```python
from build123d import *

# Parameters (mm, degrees)
SKETCH1_W           = 271.78
SKETCH1_H           = 121.92
SKETCH1_R           = 2.54
BOSS_EXTRUDE1_DEPTH = 5.08
FILLET1_R           = 6.35
SKETCH3_W           = 17.4625
SKETCH3_H           = 5.08
CUT_EXTRUDE2_DEPTH  = 7.62
FILLET2_R           = 11.43


with BuildPart() as part:
    # Sketch1 → Boss-Extrude1 (new body)
    with BuildSketch(Plane(origin=(0, 0, 0), x_dir=(1, 0, 0), z_dir=(0, 1, 0))):
        Rectangle(SKETCH1_W, SKETCH1_H)
        with Locations((-50.8, -38.1)):
            Circle(SKETCH1_R, mode=Mode.SUBTRACT)
        Polygon((-125.73, 42.241214341), (-94.577104423, 0), (-125.73, -42.241214341), align=None, mode=Mode.SUBTRACT)
        Polygon((-88.265, -8.558785659), (-57.112104423, -50.8), (-119.417895577, -50.8), align=None, mode=Mode.SUBTRACT)
        Polygon((-55.88, -35.353078748), (-81.952895577, 0), (-55.88, 35.353078748), align=None, mode=Mode.SUBTRACT)
        Polygon((-35.524026052, -50.8), (37.465, -8.791927452), (110.454026052, -50.8), align=None, mode=Mode.SUBTRACT)
        Polygon((22.189026052, 0), (-45.72, -39.084331541), (-45.72, 39.084331541), align=None, mode=Mode.SUBTRACT)
        Polygon((-57.112104423, 50.8), (-88.265, 8.558785659), (-119.417895577, 50.8), align=None, mode=Mode.SUBTRACT)
        with Locations((-50.8, 38.1)):
            Circle(SKETCH1_R, mode=Mode.SUBTRACT)
        Polygon((52.740973948, 0), (125.73, 42.008072548), (125.73, -42.008072548), align=None, mode=Mode.SUBTRACT)
        Polygon((110.454026052, 50.8), (37.465, 8.791927452), (-35.524026052, 50.8), align=None, mode=Mode.SUBTRACT)
    extrude(amount=BOSS_EXTRUDE1_DEPTH)

    # Fillet1
    fillet1_edges = [part.edges().sort_by_distance(p)[0] for p in [
        (-35.524026052, 2.54, 50.8),
        (37.465, 2.54, 8.791927452),
        (125.73, 2.54, 42.008072548),
        (125.73, 2.54, -42.008072548),
        (52.740973948, 2.54, 0),
        (-45.72, 2.54, 39.084331541),
        (22.189026052, 2.54, 0),
        (-45.72, 2.54, -39.084331541),
        (-35.524026052, 2.54, -50.8),
        (37.465, 2.54, -8.791927452),
        (-125.73, 2.54, -42.241214341),
        (-125.73, 2.54, 42.241214341),
        (-94.577104423, 2.54, 0),
        (-57.112104423, 2.54, -50.8),
        (-119.417895577, 2.54, -50.8),
        (-88.265, 2.54, -8.558785659),
        (-119.417895577, 2.54, 50.8),
        (-57.112104423, 2.54, 50.8),
        (-88.265, 2.54, 8.558785659),
        (-55.88, 2.54, 35.353078748),
        (-55.88, 2.54, -35.353078748),
        (-81.952895577, 2.54, 0),
    ]]
    fillet(fillet1_edges, radius=FILLET1_R)

    # Sketch3 → Cut-Extrude2 (cut)
    with BuildSketch(Plane(origin=(0, 5.08, 0), x_dir=(1, 0, 0), z_dir=(0, 1, 0))):
        with Locations((92.23375, 58.42)):
            Rectangle(SKETCH3_W, SKETCH3_H)
        with Locations((127.15875, 58.42)):
            Rectangle(SKETCH3_W, SKETCH3_H)
        with Locations((92.23375, -58.42)):
            Rectangle(SKETCH3_W, SKETCH3_H)
        with Locations((127.15875, -58.42)):
            Rectangle(SKETCH3_W, SKETCH3_H)
    extrude(amount=-CUT_EXTRUDE2_DEPTH, mode=Mode.SUBTRACT)

    # Fillet2
    fillet2_edges = [part.edges().sort_by_distance(p)[0] for p in [
        (110.454026052, 2.54, 50.8),
        (110.454026052, 2.54, -50.8),
    ]]
    fillet(fillet2_edges, radius=FILLET2_R)


solid = part.part
```
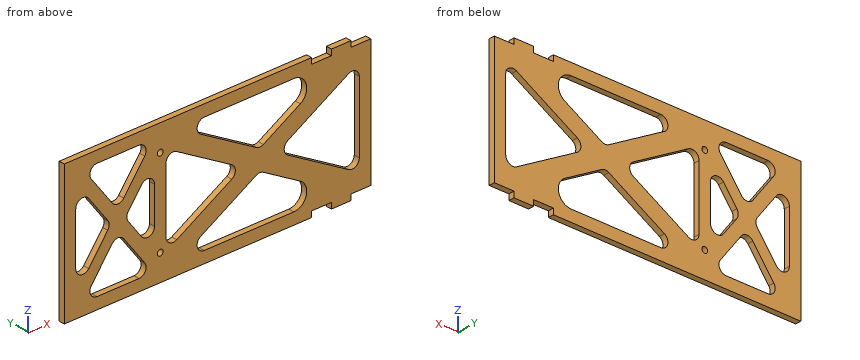
Design review of the part built by this model. Coordinates are the model's own, in mm. Coordinates: 2 decimals unless noted, no trailing zeros. Order: outer loops, then holes, each group sorted by start corner. A loop starts at its lowest first (then second) coordinate and runs counter-clockwise, first axis right, second up. Notation, with made-up numbers: (34.25, -21.75) -> (88.25, -21.75) arc R20 cw to (88.25, 15.25) -> close; hole circle Ø8 at (-6.5, 53.25). An arc over 180 degrees is marked (long way). One line per item, written item: value. Start each with the question number.
Q1. Take a section at B-B, the plane z = 0.5. State the section outline as (x, y) points, then the cut area to 3 significant figures.
Q2. Take a section at A-A, the plane x = -50.8. State the section outline as (y, z) points.
Q3. For probe 1 along Z at (x, y) = (-50.8, 1.85); probe 2 along X at (y, z) = (2.55, 29.5); probe 3 along Z at (x, y) = (-109.5, 0.35), list the stretches that pass through material, from the lowest coordinate up.
Q4. Insertion check: pin 1 Ø1.5 at (y, z) = (2, 58.5) entering from +X; pin 2 Ø1.5 at (x, y) = (124.5, 3) entering from -Z. Each pin has a flat end and moves straight along its axis. Give the tip position at first contact, or say it passes through.
Q5. Take a section at C-C, the plane y = 1.85. Give the number of separate pieces and of enclosed holes in the cut face, then the cut area to 3 significant figures.
Values follow:
1. outline: (-135.89, 0) -> (-125.73, 0) -> (-125.73, 5.08) -> (-135.89, 5.08) -> close; (-96.14, 0) -> (-80.39, 0) -> (-80.39, 5.08) -> (-96.14, 5.08) -> close; (-55.88, 0) -> (-45.72, 0) -> (-45.72, 5.08) -> (-55.88, 5.08) -> close; (15.79, 0) -> (59.14, 0) -> (59.14, 5.08) -> (15.79, 5.08) -> close; (125.73, 0) -> (135.89, 0) -> (135.89, 5.08) -> (125.73, 5.08) -> close
1. area: 455 mm2
2. outline: (0, -60.96) -> (5.08, -60.96) -> (5.08, -40.64) -> (0, -40.64) -> close; (0, -35.56) -> (5.08, -35.56) -> (5.08, 35.56) -> (0, 35.56) -> close; (0, 40.64) -> (5.08, 40.64) -> (5.08, 60.96) -> (0, 60.96) -> close
3. probe 1: z = -60.96 to -40.64, -35.56 to 35.56, 40.64 to 60.96
3. probe 2: x = -135.89 to -103.71, -72.82 to -45.56, -29.07 to 1.48, 73.44 to 104, 125.73 to 135.89
3. probe 3: z = -60.96 to -50.22, -37.35 to -20.23, 20.23 to 37.35, 50.22 to 60.96
4. pin 1: stops at x = 118.43
4. pin 2: stops at z = -55.88
5. separate pieces: 1
5. enclosed holes: 10
5. area: 17,500 mm2
